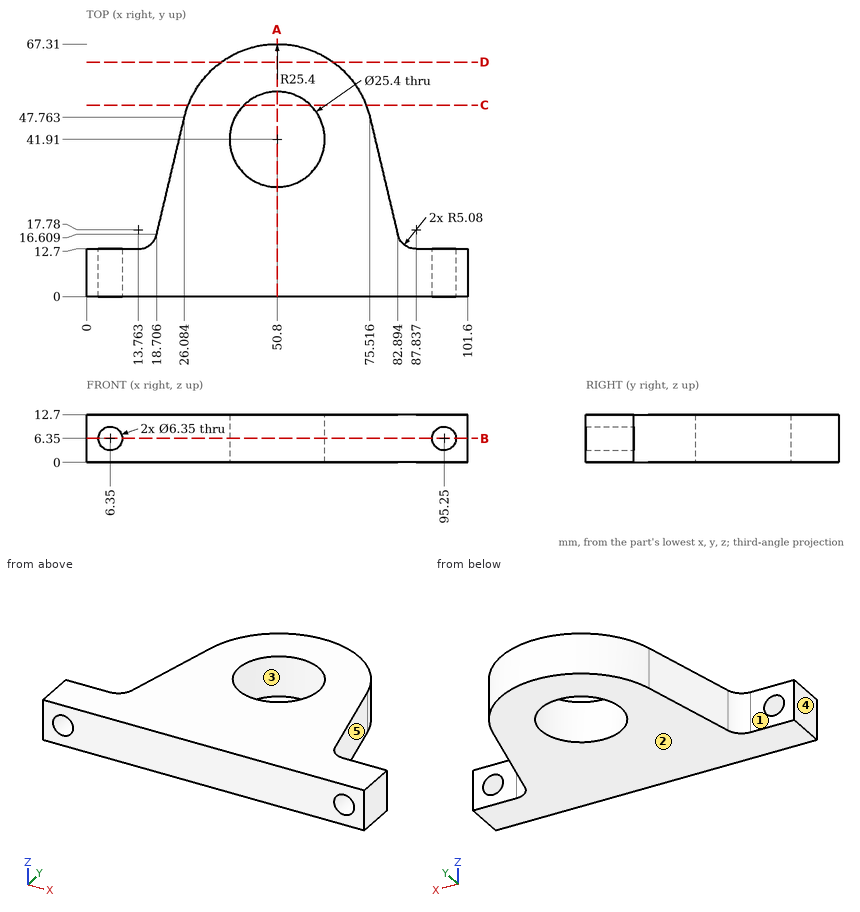
Input: dimensioned drawing with shaded views. Units: mm. Origin: part minimum x, y, z. A direction names the side the tool comes from. Give positions to 0.01 mm unless a question says otherwise; leave off trailing zeros. Write each loop counter-clockwise with the first axis right and the second up, starting at its lowest first coordinate (ties: lowest second). Pieces come first, ordered by that corner, then holes. Notation, with made-up numbers: M 10,8.5 L 66,8.5 A7 cw 66,18.5 Z; hole C 44,32.25 d2. An arc over 180 degrees is marked long. Write item = value, one per line. Start each with the question number.
1) Material intervals for line 1 along X through (y, z) = (7.25, 6.35) (1 decimal); line 2 along Z through (x, y) = (6, 3) (1 decimal); line 3 along X through (y, z) = (44.5, 5.75), sorted ascending. Write a range as [from, to].
2) Draft query along X for the marked faces 3, 4 and 5. Return one class per face: +X half, -X half, draft (parallel to the pull), parting line (faces both ways), or undercut.
3) Cut plane B-B on z = 6.35. Return the cut outline in (x, y) (1 decimal).
4) Cut plane D-D on y = 62.5. Return the cut outline in (x, z).
5) Cut plane C-C on y = 51. Return the cut outline in (x, z).
6) Cut plane A-A on x = 50.8. Return the cut outline in (y, z), then the cut area to 3 significant figures.
7) First-contact query: pin 1 Ø3 at (x, y) = (60, 53.5) entering from -Z; pin 2 Ø6 at (y, z) = (25.5, 4) entering from -X; pin 3 Ø1.5 at (y, z) = (43, 4) entering from +X; pin 4 Ø1.5 at (x, z) = (38, 2) entering from +Y. Flat tips, straight axial feed; report the tip coordinate or a pass-through.
8) Reachability of the marked faces 1 and 2 from +Z, -Z, +X, -X, +Y, -Y: full face, straight path, thin tool, end or side. Return the list, or none.
Solved:
q1.line_1 = [0, 3.2], [9.5, 92.1], [98.4, 101.6]
q1.line_2 = [0, 3.2], [9.5, 12.7]
q1.line_3 = [25.31, 38.37], [63.23, 76.29]
q2.face_3 = undercut
q2.face_4 = -X half
q2.face_5 = +X half
q3.outline = M 0,0 L 3.2,0 L 3.2,12.7 L 0,12.7 Z; M 9.5,0 L 92.1,0 L 92.1,12.7 L 87.8,12.7 A5.1 cw 82.9,16.6 L 75.5,47.8 A25.4 ccw 26.1,47.8 L 18.7,16.6 A5.1 cw 13.8,12.7 L 9.5,12.7 Z; M 98.4,0 L 101.6,0 L 101.6,12.7 L 98.4,12.7 Z; hole C 50.8,41.9 d25.4
q4.outline = M 35.93,0 L 65.67,0 L 65.67,12.7 L 35.93,12.7 Z
q5.outline = M 27.08,0 L 41.93,0 L 41.93,12.7 L 27.08,12.7 Z; M 59.67,0 L 74.52,0 L 74.52,12.7 L 59.67,12.7 Z
q6.outline = M 0,0 L 29.21,0 L 29.21,12.7 L 0,12.7 Z; M 54.61,0 L 67.31,0 L 67.31,12.7 L 54.61,12.7 Z
q6.area = 532 mm2
q7.pin_1 = 0
q7.pin_2 = 20.1
q7.pin_3 = 76.82
q7.pin_4 = 64.27
q8.face_1 = +Z, -Z, -X, +Y
q8.face_2 = -Z, +X, -X, +Y, -Y
